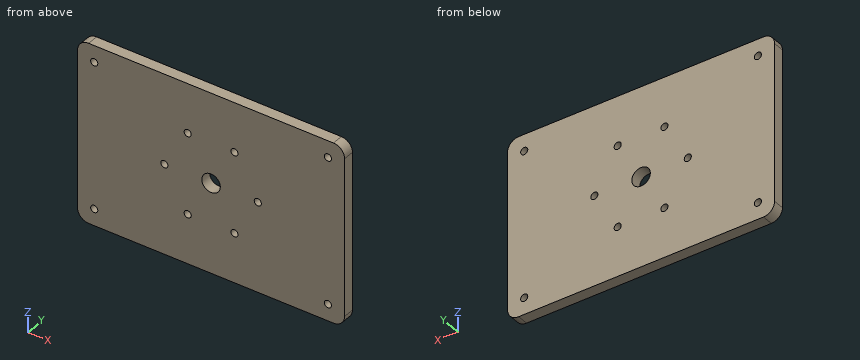
```python
from build123d import *

# Parameters (mm, degrees)
SKETCH1_W           = 120
SKETCH1_H           = 80.79
SKETCH1_R           = 1.6
SKETCH1_R_2         = 4.15
BOSS_EXTRUDE1_DEPTH = 5
SKETCH2_R           = 1.6
CUT_EXTRUDE1_DEPTH  = 6
FILLET1_R           = 5


with BuildPart() as part:
    # Sketch1 → Boss-Extrude1 (new body)
    with BuildSketch(Plane(origin=(0, 0, 0), x_dir=(1, 0, 0), z_dir=(0, 1, 0))):
        with Locations((60, 40.395)):
            Rectangle(SKETCH1_W, SKETCH1_H)
        with Locations((39, 40.395)):
            Circle(SKETCH1_R, mode=Mode.SUBTRACT)
        with Locations((49.5, 58.581533479)):
            Circle(SKETCH1_R, mode=Mode.SUBTRACT)
        with Locations((70.5, 58.581533479)):
            Circle(SKETCH1_R, mode=Mode.SUBTRACT)
        with Locations((81, 40.395)):
            Circle(SKETCH1_R, mode=Mode.SUBTRACT)
        with Locations((60, 40.395)):
            Circle(SKETCH1_R_2, mode=Mode.SUBTRACT)
        with Locations((70.5, 22.208466521)):
            Circle(SKETCH1_R, mode=Mode.SUBTRACT)
        with Locations((49.5, 22.208466521)):
            Circle(SKETCH1_R, mode=Mode.SUBTRACT)
    extrude(amount=BOSS_EXTRUDE1_DEPTH)

    # Sketch2 → Cut-Extrude1 (cut, through all)
    with BuildSketch(Plane(origin=(0, 5, 0), x_dir=(1, 0, 0), z_dir=(0, 1, 0))):
        with Locations((7.5, 73.29)):
            Circle(SKETCH2_R)
        with Locations((7.5, 7.5)):
            Circle(SKETCH2_R)
        with Locations((112.5, 73.29)):
            Circle(SKETCH2_R)
        with Locations((112.5, 7.5)):
            Circle(SKETCH2_R)
    extrude(amount=-CUT_EXTRUDE1_DEPTH, mode=Mode.SUBTRACT)

    # Fillet1
    fillet1_edges = [part.edges().sort_by_distance(p)[0] for p in [
        (0, 2.5, -80.79),
        (120, 2.5, -80.79),
        (120, 2.5, 0),
        (0, 2.5, 0),
    ]]
    fillet(fillet1_edges, radius=FILLET1_R)


solid = part.part
```
Part model, mm, in its own coordinate system. Give positions to 0.01 mm unless a question says otherwise; leave off trailing zeros. Order: outer loops, then holes, each group sorted by start corner. A loop starts at its lowest first (then second) coordinate and runs counter-clockwise, first axis right, second up. Notation, with made-up numbers: M 76,-39.75 L 135,-39.75 A30 cw 135,-7.75 Z; hole C 82,76 d3. An arc over 180 degrees is marked long. Use a Markdown table: item, result. Add a question column.
(1) Saw through at C-C, the plane y = 2.15. Give the number of separate pieces and of enclosed holes in the cut face, and give its area (3 significant figures).
(2) Saw through at A-A, the plane x = 60. Give the cut face in (y, z) (3 decimals).
(3) Saw through at D-D, the plane x = 39. Give the cut face in (y, z) (3 decimals), and give its area (3 significant figures).
(4) Saw through at B-B, the plane z = -7.5. Give the cut face in (x, y), and give its area (3 significant figures).
(5) Probe line 1 along X through (y, z) = (3.5, -7.5); line 2 along Z through (x, y) = (60, 2.2) (3 decimals); line 3 along Z through (x, y) = (70, 4). List the from-to ranges inside material, lowest first. Write a range as [from, to].
Answer key:
| question | item | result |
|---|---|---|
| 1 | separate pieces | 1 |
| 1 | enclosed holes | 11 |
| 1 | area | 9,540 mm^2 |
| 2 | outline | M 0,-80.79 L 5,-80.79 L 5,-44.545 L 0,-44.545 Z; M 0,-36.245 L 5,-36.245 L 5,0 L 0,0 Z |
| 3 | outline | M 0,-80.79 L 5,-80.79 L 5,-41.995 L 0,-41.995 Z; M 0,-38.795 L 5,-38.795 L 5,0 L 0,0 Z |
| 3 | area | 388 mm^2 |
| 4 | outline | M 0,0 L 5.9,0 L 5.9,5 L 0,5 Z; M 9.1,0 L 110.9,0 L 110.9,5 L 9.1,5 Z; M 114.1,0 L 120,0 L 120,5 L 114.1,5 Z |
| 4 | area | 568 mm^2 |
| 5 | line 1 | [0, 5.9], [9.1, 110.9], [114.1, 120] |
| 5 | line 2 | [-80.79, -44.545], [-36.245, 0] |
| 5 | line 3 | [-80.79, -60.1], [-57.06, -23.73], [-20.69, 0] |
